Verification items for this drawing (mm, ordinates from the low corner). A direction names the side the tool comes from. Give positions to 0.01 mm unless a question says otherwise; leave off trailing zeros. Loops run counter-clockwise (first coordinate to the right, second up) from the corner with the lowest first, then second, coordinate; pieces in that order, holes last. Notation, with made-up numbers: (58, 45.5) -> (107, 45.5) arc R33 cw to (107, 78.5) -> close; hole circle Ø10 at (7.5, 71.5). An arc over 180 degrees is marked (long way). Write item = value, one per line.
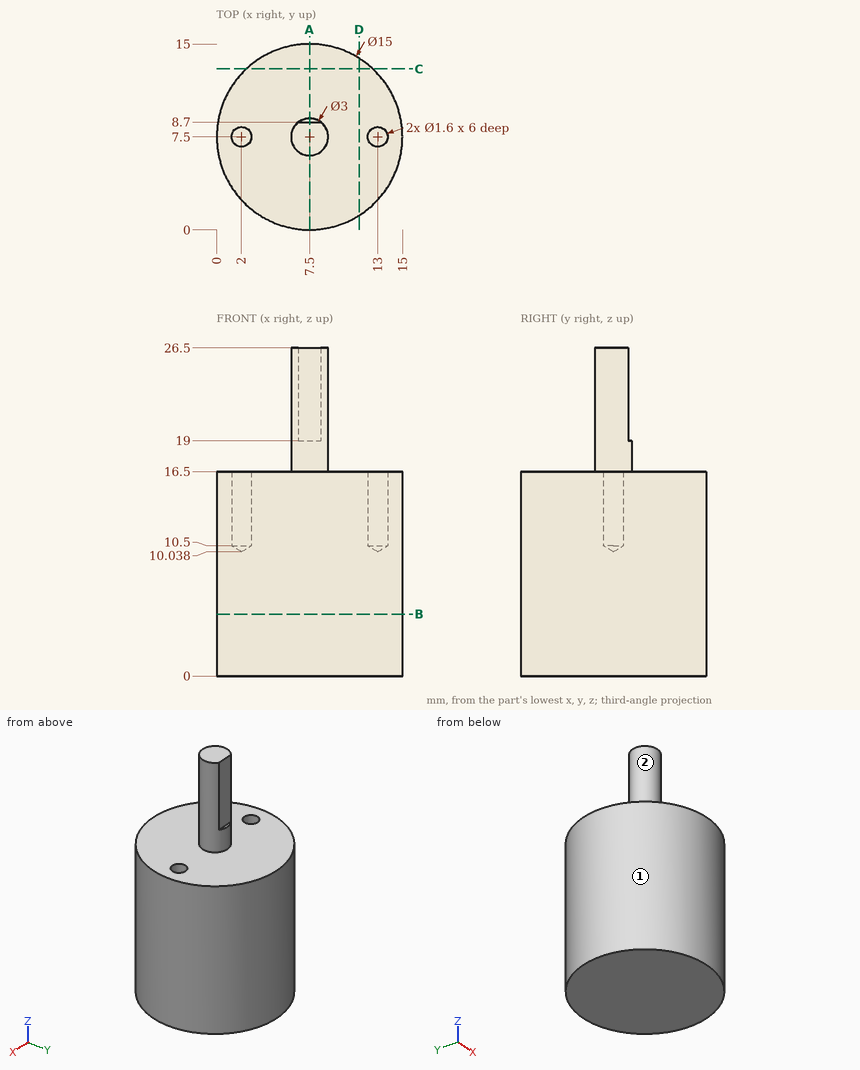
Item 1: Section check C-C, the plane y = 13. Record the cut outline in (x, z).
Answer:
outline = (2.4, 0) -> (12.6, 0) -> (12.6, 16.5) -> (2.4, 16.5) -> close
Item 2: Section check B-B, the plane z = 5. Record the cut outline in (x, y).
Answer:
outline = circle Ø15 at (7.5, 7.5)
Item 3: Gauge pin test, flat ends, axial feed: pin 1 (2 mm diameter, centred on x = 13, z = 16, fed in from -Y); pin 2 (1.5 mm diameter, centred on y = 9, z = 23, fed in from +X); pin 3 (2 mm diameter, centred on x = 7.5, z = 22, fed in from +Y). Record the tip position at first contact, or that the pin passes through.
Answer:
pin_1 = 1.5
pin_2 = 8.8
pin_3 = 8.7
Item 4: Tool access check on the marked faces 1 and 2. Record the directions out of +Z, -Z, +X, -X, +Y, -Y that give a thin tool (end or side, any length) a straight path to the whole face; none if there is none.
Answer:
face_1 = +Z, -Z
face_2 = +Z
Item 5: Section check A-A, the plane x = 7.5. Record the cut outline in (y, z), plus the area to 3 significant figures.
Answer:
outline = (0, 0) -> (15, 0) -> (15, 16.5) -> (9, 16.5) -> (9, 19) -> (8.7, 19) -> (8.7, 26.5) -> (6, 26.5) -> (6, 16.5) -> (0, 16.5) -> close
area = 275 mm^2
Item 6: Section check D-D, the plane x = 11.5. Record the cut outline in (y, z), plus the area to 3 significant figures.
Answer:
outline = (1.16, 0) -> (13.84, 0) -> (13.84, 16.5) -> (1.16, 16.5) -> close
area = 209 mm^2
Item 7: Thickness scan on L1, parallel to Z at x = 5.75, y = 2; L2, parallel to Y at x = 2, z = 14.1; L3, parallel to Y at x = 12.75, z = 13.5. Record the ranges inside material, lowest first. Write a range as [from, to].
Answer:
L1 = [0, 16.5]
L2 = [2.4, 6.7], [8.3, 12.6]
L3 = [2.14, 6.74], [8.26, 12.86]
